```python
from build123d import *

# Parameters (mm, degrees)
SKETCH1_R           = 3.96875
SKETCH1_R_2         = 2.286
BOSS_EXTRUDE1_DEPTH = 6.35


with BuildPart() as part:
    # Sketch1 → Boss-Extrude1 (new, symmetric)
    with BuildSketch(Plane(origin=(0, 0, 0), x_dir=(1, 0, 0), z_dir=(0, 1, 0))):
        Polygon((25.4, 22.225), (45.823533094, 12.53282474), (45.719315816, -0.166747645), (25.4, 0), (0, 0), (0, 22.225), align=None)
        with Locations(Location((39.422580786, 6.35, 0), (0, 0, 270))):
            Circle(SKETCH1_R, mode=Mode.SUBTRACT)
        with Locations(Location((6.35, 4.7625, 0), (0, 0, 270))):
            Circle(SKETCH1_R_2, mode=Mode.SUBTRACT)
        with Locations(Location((19.05, 4.7625, 0), (0, 0, 270))):
            Circle(SKETCH1_R_2, mode=Mode.SUBTRACT)
        with Locations(Location((19.05, 17.4625, 0), (0, 0, 270))):
            Circle(SKETCH1_R_2, mode=Mode.SUBTRACT)
        with Locations(Location((6.35, 17.4625, 0), (0, 0, 270))):
            Circle(SKETCH1_R_2, mode=Mode.SUBTRACT)
    extrude(amount=BOSS_EXTRUDE1_DEPTH, both=True)


solid = part.part
```
For this review, take the finished solid that the model builds, in its own axes (mm). A direction names the side the tool comes from. Round coordinates to 2 decimals unless told otherwise and drop trailing zeros. Loops run counter-clockwise (first coordinate to the right, second up) from the corner with the lowest first, then second, coordinate; pieces in that order, holes last.
Q1. Machinability: for faces 1 (the face through (0, 0, -11)), 2 (the face through (13, 0, 0)), which of the approach directions +Z, -Z, +X, -X, +Y, -Y give a long, thin tool a straight path to every point of the face, cutting with its end or side? Answer none if there is none.
Result sheet:
face 1: +Z, -Z, -X, +Y, -Y
face 2: +Z, -X, +Y, -Y
Q2. Mouldability with a two-part tool opening along X and no side actions: class faces 3 (the face through (35.469, 0.089, -17.447)), 4 (the face through (37.01, -0.09, -9.5)), 5 (the face through (23, 6.35, -11)) as +X half, -X half, draft (parallel to the pull), parting line (faces both ways), or undercut.
Result sheet:
face 3: +X half
face 4: undercut
face 5: draft
Q3. To check wall thickness, follow line 1 along X through (y, z) = (-1.25, -3.5); line 2 along X through (y, z) = (-2.25, -18.75); line 3 along X through (y, z) = (-1.75, -4.75). State the ranges of each line that lie inside material, in increasing order.
Result sheet:
line 1: x = 0 to 4.44, 8.26 to 17.14, 20.96 to 36.66, 42.18 to 45.75
line 2: x = 0 to 4.46, 8.24 to 17.16, 20.94 to 32.72
line 3: x = 0 to 4.06, 8.64 to 16.76, 21.34 to 35.79, 43.05 to 45.76
Q4. Insertion check: pin 1 Ø6.5 at (x, y) = (14.5, 2.5) entering from +Z; pin 2 Ø6 at (x, y) = (32.5, 1) entering from -Z; pin 3 Ø1.5 at (y, z) = (2, -14) entering from +X. Each pin has a flat end and moves straight along its axis. Give the tip position at first contact, or say it passes through.
Result sheet:
pin 1: stops at z = 0
pin 2: stops at z = -20.28
pin 3: stops at x = 44.31
Q5. Add section D-D on z = -13.5. Write out the cut boundary in (x, y).
Result sheet:
outline: (0, -6.35) - (43.79, -6.35) - (43.79, 6.35) - (0, 6.35) - close
Q6. Add section B-B on z = -6.35. Write out the cut boundary in (x, y), plus the area to 3 significant figures.
Result sheet:
outline: (0, -6.35) - (4.71, -6.35) - (4.71, 6.35) - (0, 6.35) - close; (7.99, -6.35) - (17.41, -6.35) - (17.41, 6.35) - (7.99, 6.35) - close; (20.69, -6.35) - (35.45, -6.35) - (35.45, 6.35) - (20.69, 6.35) - close; (43.39, -6.35) - (45.77, -6.35) - (45.77, 6.35) - (43.39, 6.35) - close
area: 397 mm2
Q7. Add section A-A on x = 6.35. Give the number of separate pieces and of enclosed holes in the cut face, plus the area to 3 significant figures.
Result sheet:
separate pieces: 3
enclosed holes: 0
area: 166 mm2
